```python
from build123d import *

# Parameters (mm, degrees)
SKETCH1_W                       = 25
SKETCH1_H                       = 25
BOSS_EXTRUDE1_DEPTH             = 152.4
CUT_EXTRUDE1_REACH              = 47
SKETCH3_R                       = 2.38125
SKETCH4_R                       = 1
CUT_EXTRUDE2_DEPTH              = 10
TAP_DRILL_FOR_M3X0_5_TAP1_D     = 2.5
TAP_DRILL_FOR_M3X0_5_TAP1_DEPTH = 15
TAP_DRILL_FOR_M3X0_5_TAP1_TIP   = 0.751075774


with BuildPart() as part:
    # Sketch1 → Boss-Extrude1 (new body)
    with BuildSketch(Plane(origin=(0, 0, 0), x_dir=(1, 0, 0), z_dir=(0, 1, 0))):
        Rectangle(SKETCH1_W, SKETCH1_H)
    extrude(amount=-BOSS_EXTRUDE1_DEPTH)

    # Sketch2 → Revolve1 (revolve)
    with BuildSketch(Plane.XY):
        Polygon((12.5, -137.4), (32.5, -152.4), (12.5, -152.4), align=None)
    revolve(axis=Axis((0, -152.4, 0), (0, 1, 0)))

    # Sketch3 → Cut-Extrude1 (cut, up to next)
    with BuildSketch(Plane.XY.offset(12.5), mode=Mode.PRIVATE) as cut_extrude1_sk1:
        Circle(SKETCH3_R)
    cut_extrude1_tool1 = extrude(cut_extrude1_sk1.sketch, amount=-CUT_EXTRUDE1_REACH, mode=Mode.PRIVATE) & part.part
    add(cut_extrude1_tool1.solids().sort_by_distance((0, 0, 12.5))[0], mode=Mode.SUBTRACT)

    # Sketch4 → Cut-Extrude2 (cut)
    with BuildSketch(Plane(origin=(0, 0, 0), x_dir=(1, 0, 0), z_dir=(0, 1, 0))):
        with Locations((-6.8, 5)):
            Circle(SKETCH4_R)
        with Locations((6.8, 5)):
            Circle(SKETCH4_R)
        with Locations((6.8, -5)):
            Circle(SKETCH4_R)
        with Locations((-6.8, -5)):
            Circle(SKETCH4_R)
    extrude(amount=-CUT_EXTRUDE2_DEPTH, mode=Mode.SUBTRACT)

    # Tap Drill for M3x0.5 Tap1
    with Locations(Plane(origin=(0, 0, 0), x_dir=(1, 0, 0), z_dir=(0, 1, 0))):
        with Locations((-6.8, -5), (-6.8, 5), (6.8, 5), (6.8, -5)):
            Hole(TAP_DRILL_FOR_M3X0_5_TAP1_D / 2, depth=TAP_DRILL_FOR_M3X0_5_TAP1_DEPTH)
            with Locations((0, 0, -(TAP_DRILL_FOR_M3X0_5_TAP1_DEPTH + TAP_DRILL_FOR_M3X0_5_TAP1_TIP / 2))):  # 118° drill point
                Cone(0, TAP_DRILL_FOR_M3X0_5_TAP1_D / 2, TAP_DRILL_FOR_M3X0_5_TAP1_TIP, mode=Mode.SUBTRACT)


solid = part.part
```
Work out the finished part from the listing and answer in its coordinate system (mm). Give positions to 0.01 mm unless a question says otherwise; leave off trailing zeros. Loops run counter-clockwise (first coordinate to the right, second up) from the corner with the lowest first, then second, coordinate; pieces in that order, holes last. Notation, with made-up numbers: (-25, 16.5) -> (14, 16.5) arc R30 ccw to (14, 40.5) -> close; hole circle Ø4 at (-19, -19.5). An arc over 180 degrees is marked (long way). One line per question, with ' | ' between items. Start each with the question number.
1) Section A-A, the plane y = -9 is taken. Determine the outline of the cut face in (x, z), then the cut area to 3 significant figures.
2) Section D-D, the plane y = -97 is taken. Determine the outline of the cut face in (x, z), then the cut area to 3 significant figures.
3) Section B-B, the plane z = 0 is taken. Determine the outline of the cut face in (x, y), then the cut area to 3 significant figures.
4) Each of these flat-tipped pins is pushed along its axis until it touches: pin 1 (20 mm diameter, centred on x = -2, y = -38.5, fed in from +Z); pin 2 (12 mm diameter, centred on x = 22, z = 2.5, fed in from +Y); pin 3 (12 mm diameter, centred on y = -36, z = -1.5, fed in from -X). Where does it stop, or does it pass through?
5) Section C-C, the plane x = 0 is taken. Determine the outline of the cut face in (y, z), then the cut area to 3 significant figures.
6) Straight lines are drawn through the part: L1, parallel to Z at x = -6.8, y = -8.5; L2, parallel to X at y = -9, z = 5; L3, parallel to X at y = -133.5, z = 5. For each, find the intervals that lie inside material, in ascending order.
Resolved:
1) outline: (-12.5, -12.5) -> (12.5, -12.5) -> (12.5, 12.5) -> (-12.5, 12.5) -> close; hole circle Ø2.5 at (-6.8, -5); hole circle Ø2.5 at (-6.8, 5); hole circle Ø2.5 at (6.8, -5); hole circle Ø2.5 at (6.8, 5) | area: 605 mm2
2) outline: (-12.5, -12.5) -> (12.5, -12.5) -> (12.5, 12.5) -> (-12.5, 12.5) -> close | area: 625 mm2
3) outline: (-32.5, -152.4) -> (32.5, -152.4) -> (12.5, -137.4) -> (12.5, 0) -> (2.38, 0) arc R2.38 cw to (-2.38, 0) -> (-12.5, 0) -> (-12.5, -137.4) -> close | area: 4,100 mm2
4) pin 1: z = 12.5 | pin 2: y = -140.13 | pin 3: x = -12.5
5) outline: (-152.4, -32.5) -> (-137.4, -12.5) -> (-2.38, -12.5) -> (-2.38, 12.5) -> (-137.4, 12.5) -> (-152.4, 32.5) -> close | area: 4,050 mm2
6) L1: -12.5 to -6.25, -3.75 to 3.75, 6.25 to 12.5 | L2: -12.5 to -8.05, -5.55 to 5.55, 8.05 to 12.5 | L3: -12.5 to 12.5
